Can you work these out from the model? Positions are in its coordinate system, mm. A direction names the side the tool comes from. Coordinates: 2 decimals unless noted, no trailing zeros. Use a Markdown table: item, result. Add a question column.
1. For pin 1 Ø2.5 at (x, z) = (2, 26) entering from +Y; pin 2 Ø2.5 at (x, z) = (2.5, 23) entering from -Y; pin 3 Ø5 at (y, z) = (5, 15.5) entering from +X, each with a flat end and sliding along its axis, tell me the tip position at first contact or that it passes through.
2. If I drill on line 1 along Y through (x, z) = (4, 31); line 2 along X through (y, z) = (-80.5, 35.5) (3 decimals); line 3 along Z through (x, y) = (17.75, -142) (3 decimals), over which ranges is the centre line in solid material (lowest first)? Write a range as from..to.
3. For faces 1 (the flat face through (4.762, 5, 19)), 2 (the flat face through (11.112, -386, 19)), 3 (the flat face through (4.762, -386, 19)), 4 (the flat face through (11.112, 5, 19)), which set-ups out of +Z, -Z, +X, -X, +Y, -Y let a thin tool reach every point of the face, with its end or its side?
```python
from build123d import *

# Parameters (mm, degrees)
F0_W     = 19.05
F0_H     = 38.1
F1_DEPTH = 381
F2_SIZE  = 3.175
F3_W     = 6.35
F3_H     = 38.1
F4_DEPTH = 9.525
F5_W     = 6.35
F5_H     = 38.1
F6_DEPTH = 9.525


with BuildPart() as f1:
    # F0 (on Front) → F1 (new body)
    with BuildSketch(Plane.XZ):
        with Locations((9.525, 19.05)):
            Rectangle(F0_W, F0_H)
    extrude(amount=F1_DEPTH)

    # F2
    f2_edges = [f1.edges().sort_by_distance(p)[0] for p in [
        (19.05, -190.5, 38.1),
        (19.05, -381, 19.05),
        (19.05, 0, 19.05),
        (19.05, -190.5, 0),
    ]]
    chamfer(f2_edges, length=F2_SIZE)

    # F3 (on face) → F4 (join)
    with BuildSketch(Plane.XZ.offset(381)):
        with Locations((7.9375, 19.05)):
            Rectangle(F3_W, F3_H)
    extrude(amount=F4_DEPTH)

    # F5 (on face) → F6 (join)
    with BuildSketch(Plane(origin=(0, 0, 0), x_dir=(-1, 0, 0), z_dir=(0, 1, 0))):
        with Locations((-7.9375, 19.05)):
            Rectangle(F5_W, F5_H)
    extrude(amount=F6_DEPTH)


solid = f1.part
```
Worked out:
| question | item | result |
|---|---|---|
| 1 | pin 1 | stops at y = 0 |
| 1 | pin 2 | stops at y = -381 |
| 1 | pin 3 | stops at x = 11.11 |
| 2 | line 1 | y = -381..0 |
| 2 | line 2 | x = 0..18.475 |
| 2 | line 3 | z = 1.875..36.225 |
| 3 | face 1 | +Z, -Z, -X, +Y |
| 3 | face 2 | +Z, -Z, +X, -Y |
| 3 | face 3 | +Z, -Z, -X, -Y |
| 3 | face 4 | +Z, -Z, +X, +Y |
